Work out the finished part from the listing and answer in its coordinate system (mm). Coordinates: 2 decimals unless noted, no trailing zeros. Order: outer loops, then holes, each group sorted by start corner. A loop starts at its lowest first (then second) coordinate and runs counter-clockwise, first axis right, second up. Notation, with made-up numbers: M 76,-15 L 81,-15 A19 ccw 81,10 Z; hole C 56,42.5 d11. An arc over 180 degrees is marked long. Write item = value, one per line. Start each with the question number.
Q1. Find section A-A on y = -1.5. Give the vertices of the cut face in (x, z).
Q2. Straight lines are drawn through the part: line 1 along Z through (x, y) = (-0.1, -3); line 2 along Z through (x, y) = (-0.7, -1.75); line 3 along X through (y, z) = (-2.5, 1.6). For each, find the intervals that lie inside material, in ascending order.
Q3. This flat-tipped pin is pushed along its axis until it touches: P1, Ø1.5, axis at y = 3, z = 1, coming from the -X side. Where does it stop, or does it pass through?
```python
from build123d import *

# Parameters (mm, degrees)
SKETCH_1_W = 2
SKETCH_1_H = 8


with BuildPart() as part:
    # 草图1 → 旋转1 (revolve)
    with BuildSketch(Plane.XY):
        with Locations((1, 0)):
            Rectangle(SKETCH_1_W, SKETCH_1_H)
    revolve(axis=Axis((0, -4, 0), (0, 1, 0)))

    # 草图2 → 切除-旋转1 (revolve, cut)
    with BuildSketch(Plane.XY):
        Polygon((1.831192009, -4), (2, -3.37), (2.1, -3.37), (2.1, -4.1), (1.831192009, -4.1), align=None)
    cut_revolve_1 = revolve(axis=Axis((0, 0, 0), (0, -1, 0)), mode=Mode.SUBTRACT)

    # 镜向1: 切除-旋转1 across plane
    add(cut_revolve_1.mirror(Plane.ZX), mode=Mode.SUBTRACT)


solid = part.part
```
Findings below:
q1.outline = C 0,0 d4
q2.line_1 = -2 to 2
q2.line_2 = -1.87 to 1.87
q2.line_3 = -1.2 to 1.2
q3.P1 = -1.98
